Answer from the drawing. Dimensions are ordinates in mm from the lowest x, y and z of the part. A direction names the side the tool comes from. Round coordinates to 2 decimals unless told otherwise and drop trailing zeros. Order: outer loops, then holes, each group sorted by start corner. A loop starts at its lowest first (then second) coordinate and runs counter-clockwise, first axis right, second up. Notation, with made-up numbers: (18.5, 38.5) -> (29.5, 38.5) arc R7 cw to (29.5, 43.5) -> close; hole circle Ø8 at (17.25, 56.25). An arc over 180 degrees is marked (long way). Use a Markdown table: item, result. Add a question column.
1. Section A-A, the plane z = 1.5 is taken. Give the vertices of the cut face in (x, y), then the cut area to 3 significant figures.
2. Consider L1, parallel to X at y = 2.4, z = 0.9; L2, parallel to X at y = 1.85, z = 1.65; L3, parallel to Y at x = 4.25, z = 1.3. Determine where each line is inside the solid, lowest interval first. Write a range as [from, to].
3. Section C-C, the plane x = 2.25 is taken. Give the vertices of the cut face in (y, z).
4. Section B-B, the plane y = 1.5 is taken. Give the vertices of the cut face in (x, z).
5. Given pin 1 (1.5 mm diameter, centred on x = 5, y = 1.5, fed in from +Z); pin 2 (1.5 mm diameter, centred on y = 0.5, z = 2, fed in from -X); pin 3 (1 mm diameter, centred on x = 2, z = 2, fed in from -Y), each flat-ended and moving along its own axis, determine where each tip first touches the part or whether it passes through.
6. For the marked faces 1 and 2, determine the directions among +Z, -Z, +X, -X, +Y, -Y from which every point of the face is accessible in a straight line to the end or side of a thin tool.
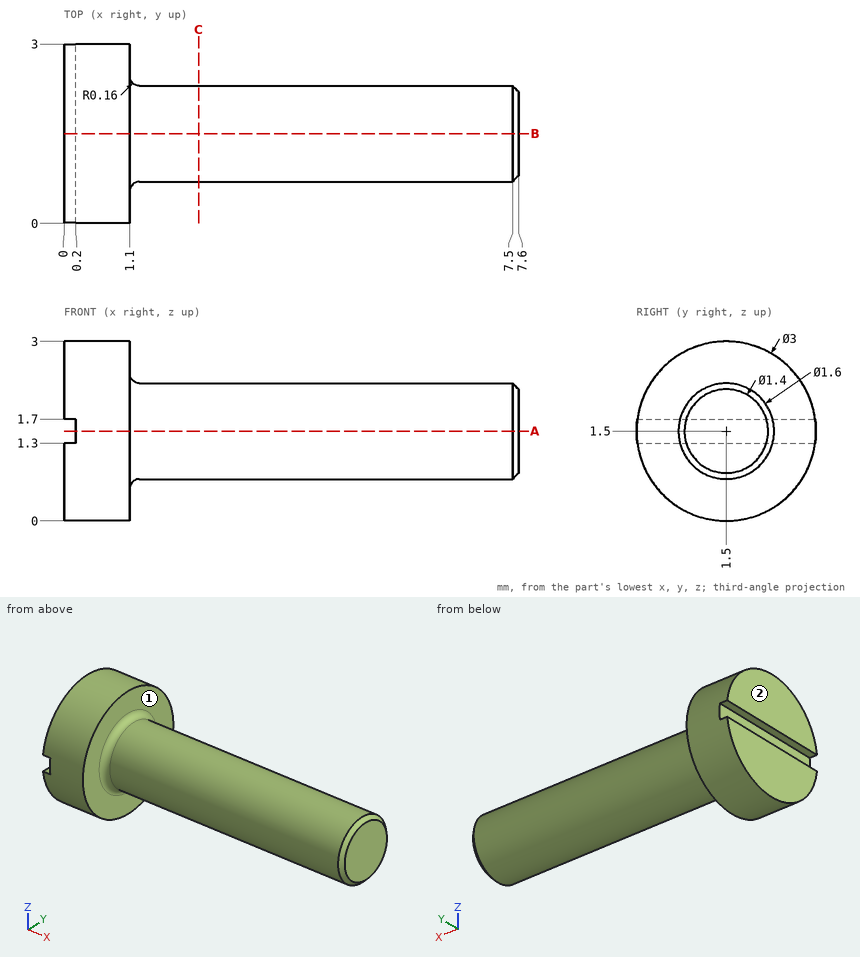
Verdict:
| question | item | result |
|---|---|---|
| 1 | outline | (0.2, 0) -> (1.1, 0) -> (1.1, 0.54) arc R0.16 cw to (1.26, 0.7) -> (7.5, 0.7) -> (7.6, 0.8) -> (7.6, 2.2) -> (7.5, 2.3) -> (1.26, 2.3) arc R0.16 cw to (1.1, 2.46) -> (1.1, 3) -> (0.2, 3) -> close |
| 1 | area | 13.1 mm2 |
| 2 | L1 | x = [0, 1.1] |
| 2 | L2 | x = [0.2, 7.6] |
| 2 | L3 | y = [0.73, 2.27] |
| 3 | outline | circle Ø1.6 at (1.5, 1.5) |
| 4 | outline | (0, 0) -> (1.1, 0) -> (1.1, 0.54) arc R0.16 cw to (1.26, 0.7) -> (7.5, 0.7) -> (7.6, 0.8) -> (7.6, 2.2) -> (7.5, 2.3) -> (1.26, 2.3) arc R0.16 cw to (1.1, 2.46) -> (1.1, 3) -> (0, 3) -> (0, 1.7) -> (0.2, 1.7) -> (0.2, 1.3) -> (0, 1.3) -> close |
| 5 | pin 1 | stops at z = 2.3 |
| 5 | pin 2 | stops at x = 0 |
| 5 | pin 3 | stops at y = 0.7 |
| 6 | face 1 | +X |
| 6 | face 2 | +Z, -Z, -X, +Y, -Y |
